CAD build for the part. Positions are in the model's coordinates, mm. A direction names the side the tool comes from. Give positions to 0.01 mm unless a question says otherwise; leave off trailing zeros. Loops run counter-clockwise (first coordinate to the right, second up) from the corner with the lowest first, then second, coordinate; pieces in that order, holes last.
Item 1: Saw through at C-C on y = -41. Give the cut face in (x, z), plus the area to 3 significant figures.
Item 2: Saw through at D-D on y = -5. Give the cut face in (x, z).
Item 3: Which spindle directions (+Z, -Z, +X, -X, +Y, -Y) get a long thin tool onto all of the face, cutting with end or side? Do faces 5 (the flat face through (0, -46, 2)), 6 (the flat face through (-30, -33, 2)). Say none if no direction does.
Item 4: Drop a flat-ended pin along its axis: P1, Ø2.5, axis at y = -38, z = 2.5, coming from the -X side. Give the stop position or say it passes through.
Item 5: Saw through at B-B on z = 4. Give the number of separate pieces and of enclosed holes in the cut face, plus the area to 3 significant figures.
Item 6: Mould opens along Y. For faces 1 (the flat face through (-9, 12, 2)), 2 (the cylindrical face through (-24.325, -42.464, 2.535)), 3 (the cylindrical face through (-35.703, -6.014, 2.535)), 4 (the cylindrical face through (-25.5, -4.93, 2.54)) say: released by +Y, released by -Y, zero draft, split by the parting line, or undercut.
Item 7: Probe probe 1 along Y at (x, z) = (24, 3.5); probe 2 along Y at (x, z) = (0, 3.5); probe 3 along X at (y, z) = (-42, 0.6). List the from-to ranges inside material, lowest first.
Item 8: Saw through at A-A on x = 0. Give the cut face in (y, z).
from build123d import *

# Parameters (mm, degrees)
SKETCH_1_R             = 2.5
EXTRUDE_1_DEPTH        = 5
CUT_EXTRUDE_1_REACH    = 74.643
SKETCH_2_R             = 1.5
PATTERN_LINEAR_1_COUNT = 5
PATTERN_LINEAR_1_PITCH = 12
FILLET_1_R             = 20


with BuildPart() as part:
    # Sketch 1 → Extrude 1 (new body)
    with BuildSketch(Plane.XY):
        with BuildLine():
            Line((-30, 0), (-30, -46))
            Line((-30, -46), (30, -46))
            Line((30, -46), (30, 0))
            Line((30, 0), (30, 12))
            Line((30, 12), (-50, 12))
            ThreePointArc((-50, 12), (-56, 6), (-50, 0))
            Line((-50, 0), (-30, 0))
        make_face()
        with Locations((0, 6)):
            Circle(SKETCH_1_R, mode=Mode.SUBTRACT)
        with Locations((-50, 6)):
            Circle(SKETCH_1_R, mode=Mode.SUBTRACT)
    extrude(amount=EXTRUDE_1_DEPTH)

    # Sketch 2 → Cut-Extrude 1 (cut, up to next)
    with BuildSketch(Plane.XY.offset(5), mode=Mode.PRIVATE) as cut_extrude_1_sk1:
        with Locations((-24, -5)):
            Circle(SKETCH_2_R)
    cut_extrude_1_tool1 = extrude(cut_extrude_1_sk1.sketch, amount=-CUT_EXTRUDE_1_REACH, mode=Mode.PRIVATE) & part.part
    # Sketch 2 → Cut-Extrude 1 (cut, up to next)
    with BuildSketch(Plane.XY.offset(5), mode=Mode.PRIVATE) as cut_extrude_1_sk2:
        with Locations((-24, -41)):
            Circle(SKETCH_2_R)
    cut_extrude_1_tool2 = extrude(cut_extrude_1_sk2.sketch, amount=-CUT_EXTRUDE_1_REACH, mode=Mode.PRIVATE) & part.part
    cut_extrude_1_1 = cut_extrude_1_tool1.solids().sort_by_distance((-24, -5, 5))[0]
    add(cut_extrude_1_1, mode=Mode.SUBTRACT)
    cut_extrude_1_2 = cut_extrude_1_tool2.solids().sort_by_distance((-24, -41, 5))[0]
    add(cut_extrude_1_2, mode=Mode.SUBTRACT)
    cut_extrude_1 = cut_extrude_1_1 + cut_extrude_1_2  # Cut-Extrude 1 as one shape, for the pattern or mirror that repeats it

    # Pattern Linear 1: Cut-Extrude 1 ×5
    with Locations(*[(i * PATTERN_LINEAR_1_PITCH, 0, 0) for i in range(1, PATTERN_LINEAR_1_COUNT)]):
        add(cut_extrude_1, mode=Mode.SUBTRACT)

    # Fillet 1
    fillet_1_edges = [part.edges().sort_by_distance(p)[0] for p in [
        (-30, 0, 2.5),
    ]]
    fillet(fillet_1_edges, radius=FILLET_1_R - 0.0001)  # a hair under: the kernel refuses the full size


solid = part.part
Results below:
1. outline: (-30, 0) - (-25.5, 0) - (-25.5, 5) - (-30, 5) - close; (-22.5, 0) - (-13.5, 0) - (-13.5, 5) - (-22.5, 5) - close; (-10.5, 0) - (-1.5, 0) - (-1.5, 5) - (-10.5, 5) - close; (1.5, 0) - (10.5, 0) - (10.5, 5) - (1.5, 5) - close; (13.5, 0) - (22.5, 0) - (22.5, 5) - (13.5, 5) - close; (25.5, 0) - (30, 0) - (30, 5) - (25.5, 5) - close
1. area: 225 mm2
2. outline: (-36.77, 0) - (-25.5, 0) - (-25.5, 5) - (-36.77, 5) - close; (-22.5, 0) - (-13.5, 0) - (-13.5, 5) - (-22.5, 5) - close; (-10.5, 0) - (-1.5, 0) - (-1.5, 5) - (-10.5, 5) - close; (1.5, 0) - (10.5, 0) - (10.5, 5) - (1.5, 5) - close; (13.5, 0) - (22.5, 0) - (22.5, 5) - (13.5, 5) - close; (25.5, 0) - (30, 0) - (30, 5) - (25.5, 5) - close
3. face 5: +Z, -Z, +X, -X, -Y
3. face 6: +Z, -Z, -X, -Y
4. P1: stops at x = -30
5. separate pieces: 1
5. enclosed holes: 12
5. area: 3,750 mm2
6. face 1: released by +Y
6. face 2: undercut
6. face 3: released by -Y
6. face 4: undercut
7. probe 1: y = -46 to -42.5, -39.5 to -6.5, -3.5 to 12
7. probe 2: y = -46 to -42.5, -39.5 to -6.5, -3.5 to 3.5, 8.5 to 12
7. probe 3: x = -30 to -25.12, -22.88 to -13.12, -10.88 to -1.12, 1.12 to 10.88, 13.12 to 22.88, 25.12 to 30
8. outline: (-46, 0) - (-42.5, 0) - (-42.5, 5) - (-46, 5) - close; (-39.5, 0) - (-6.5, 0) - (-6.5, 5) - (-39.5, 5) - close; (-3.5, 0) - (3.5, 0) - (3.5, 5) - (-3.5, 5) - close; (8.5, 0) - (12, 0) - (12, 5) - (8.5, 5) - close
